Read the model definition and answer for the solid it produces. Units are mm, in the model's axes. Face numbers are marked on the shaded views. A direction names the side the tool comes from. Give positions to 0.01 mm unless a question says otherwise; leave off trailing zeros. Order: outer loops, then holes, each group sorted by start corner. A loop starts at its lowest first (then second) coordinate and runs counter-clockwise, first axis right, second up.
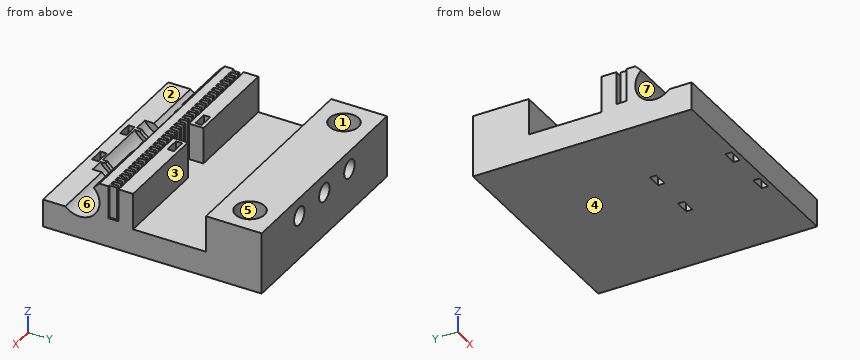
```python
from build123d import *

# Parameters (mm, degrees)
SKETCH1_W           = 60
SKETCH1_H           = 17
BOSS_EXTRUDE2_DEPTH = 60
SKETCH5_R           = 7.5
CUT_EXTRUDE3_DEPTH  = 12.5
BOSS_EXTRUDE5_START = 1
SKETCH7_R           = 7.5
SKETCH7_R_2         = 6.375
BOSS_EXTRUDE5_DEPTH = 1
SKETCH8_R           = 7.5
SKETCH8_R_2         = 6.375
BOSS_EXTRUDE6_DEPTH = 1
SKETCH3_W           = 14.616308542
SKETCH3_H           = 2.75
CUT_EXTRUDE2_DEPTH  = 87.539008545
SKETCH9_W           = 29.365083629
SKETCH9_H           = 1.75
SKETCH9_W_2         = 26.887211927
CUT_EXTRUDE4_DEPTH  = 4
SKETCH10_W          = 36.539507471
SKETCH10_H          = 1.75
SKETCH10_W_2        = 38.625095797
CUT_EXTRUDE5_DEPTH  = 4
SKETCH12_W          = 0.85
SKETCH12_H          = 2
BOSS_EXTRUDE7_DEPTH = 9
CUT_EXTRUDE6_DEPTH  = 10
SKETCH14_R          = 4
CUT_EXTRUDE7_DEPTH  = 15
SKETCH15_R          = 2.5
CUT_EXTRUDE8_DEPTH  = 15.3


with BuildPart() as part:
    # Sketch1 → Boss-Extrude2 (new body)
    with BuildSketch(Plane(origin=(0, 0, 0), x_dir=(1, 0, 0), z_dir=(0, 1, 0))):
        with Locations((30, 8.5)):
            Rectangle(SKETCH1_W, SKETCH1_H)
    extrude(amount=BOSS_EXTRUDE2_DEPTH)

    # Sketch5 → Cut-Extrude3 (cut, symmetric)
    with BuildSketch(Plane(origin=(30, 0, 0), x_dir=(0, 0, -1), z_dir=(1, 0, 0))):
        with Locations((5.5, 10)):
            Circle(SKETCH5_R)
    extrude(amount=CUT_EXTRUDE3_DEPTH, both=True, mode=Mode.SUBTRACT)

    # Sketch7 → Boss-Extrude5 (add)
    with BuildSketch(Plane(origin=(21.3, 0, 0), x_dir=(0, 0, -1), z_dir=(1, 0, 0)).offset(BOSS_EXTRUDE5_START)):
        with Locations((5.5, 10)):
            Circle(SKETCH7_R)
        with Locations((5.5, 10)):
            Circle(SKETCH7_R_2, mode=Mode.SUBTRACT)
    extrude(amount=-BOSS_EXTRUDE5_DEPTH)

    # Sketch8 → Boss-Extrude6 (add)
    with BuildSketch(Plane.ZY.offset(-38.7)):
        with Locations((-5.5, 10)):
            Circle(SKETCH8_R)
        with Locations(Location((-5.5, 10, 0), (0, 0, 180))):
            Circle(SKETCH8_R_2, mode=Mode.SUBTRACT)
    extrude(amount=BOSS_EXTRUDE6_DEPTH)

    # Sketch3 → Cut-Extrude2 (cut, through all)
    with BuildSketch(Plane(origin=(60, 0, 0), x_dir=(0, 0, -1), z_dir=(1, 0, 0))):
        with BuildLine():
            Line((0, 15.5), (-6.640665203, 15.5))
            Line((-6.640665203, 15.5), (-6.640665203, 0))
            Line((-6.640665203, 0), (0, 0))
            Line((0, 0), (9.389087297, 0))
            Line((9.389087297, 0), (9.389087297, 6.110912703))
            ThreePointArc((9.389087297, 6.110912703), (9.389087297, 13.889087297), (1.610912703, 13.889087297))
            Line((1.610912703, 13.889087297), (0, 15.5))
        make_face()
        with Locations((1.691845729, 19.325)):
            Rectangle(SKETCH3_W, SKETCH3_H)
    extrude(amount=-CUT_EXTRUDE2_DEPTH, mode=Mode.SUBTRACT)

    # Sketch9 → Cut-Extrude4 (cut)
    with BuildSketch(Plane(origin=(21.3, 0, 0), x_dir=(0, 0, -1), z_dir=(1, 0, 0))):
        with Locations((7.065771792, 2.125)):
            Rectangle(SKETCH9_W, SKETCH9_H)
        with Locations((6.15524604, 22.825)):
            Rectangle(SKETCH9_W_2, SKETCH9_H)
    extrude(amount=CUT_EXTRUDE4_DEPTH, mode=Mode.SUBTRACT)

    # Sketch10 → Cut-Extrude5 (cut)
    with BuildSketch(Plane.ZY.offset(-38.7)):
        with Locations((-12.469654385, 22.825)):
            Rectangle(SKETCH10_W, SKETCH10_H)
        with Locations((-10.676048425, 2.125)):
            Rectangle(SKETCH10_W_2, SKETCH10_H)
    extrude(amount=CUT_EXTRUDE5_DEPTH, mode=Mode.SUBTRACT)

    # Sketch12 → Boss-Extrude7 (add)
    with BuildSketch(Plane.XY.offset(-9)):
        with Locations((59.075, 18.95)):
            Rectangle(SKETCH12_W, SKETCH12_H)
        with Locations((57.075, 18.95)):
            Rectangle(SKETCH12_W, SKETCH12_H)
        with Locations((55.075, 18.95)):
            Rectangle(SKETCH12_W, SKETCH12_H)
        with Locations((53.075, 18.95)):
            Rectangle(SKETCH12_W, SKETCH12_H)
        with Locations((51.075, 18.95)):
            Rectangle(SKETCH12_W, SKETCH12_H)
        with Locations((49.075, 18.95)):
            Rectangle(SKETCH12_W, SKETCH12_H)
        with Locations((47.075, 18.95)):
            Rectangle(SKETCH12_W, SKETCH12_H)
        with Locations((45.075, 18.95)):
            Rectangle(SKETCH12_W, SKETCH12_H)
        with Locations((43.075, 18.95)):
            Rectangle(SKETCH12_W, SKETCH12_H)
        with Locations((41.075, 18.95)):
            Rectangle(SKETCH12_W, SKETCH12_H)
        with Locations((39.075, 18.95)):
            Rectangle(SKETCH12_W, SKETCH12_H)
        with Locations((37.075, 18.95)):
            Rectangle(SKETCH12_W, SKETCH12_H)
        with Locations((35.075, 18.95)):
            Rectangle(SKETCH12_W, SKETCH12_H)
        with Locations((33.075, 18.95)):
            Rectangle(SKETCH12_W, SKETCH12_H)
        with Locations((31.075, 18.95)):
            Rectangle(SKETCH12_W, SKETCH12_H)
        with Locations((29.075, 18.95)):
            Rectangle(SKETCH12_W, SKETCH12_H)
        with Locations((27.075, 18.95)):
            Rectangle(SKETCH12_W, SKETCH12_H)
        with Locations((25.075, 18.95)):
            Rectangle(SKETCH12_W, SKETCH12_H)
        with Locations((23.075, 18.95)):
            Rectangle(SKETCH12_W, SKETCH12_H)
        with Locations((21.075, 18.95)):
            Rectangle(SKETCH12_W, SKETCH12_H)
        with Locations((19.075, 18.95)):
            Rectangle(SKETCH12_W, SKETCH12_H)
        with Locations((17.075, 18.95)):
            Rectangle(SKETCH12_W, SKETCH12_H)
        with Locations((15.075, 18.95)):
            Rectangle(SKETCH12_W, SKETCH12_H)
        with Locations((13.075, 18.95)):
            Rectangle(SKETCH12_W, SKETCH12_H)
        with Locations((11.075, 18.95)):
            Rectangle(SKETCH12_W, SKETCH12_H)
        with Locations((9.075, 18.95)):
            Rectangle(SKETCH12_W, SKETCH12_H)
        with Locations((7.075, 18.95)):
            Rectangle(SKETCH12_W, SKETCH12_H)
        with Locations((5.075, 18.95)):
            Rectangle(SKETCH12_W, SKETCH12_H)
        with Locations((3.075, 18.95)):
            Rectangle(SKETCH12_W, SKETCH12_H)
        with Locations((1.075, 18.95)):
            Rectangle(SKETCH12_W, SKETCH12_H)
    extrude(amount=BOSS_EXTRUDE7_DEPTH)

    # Sketch13 → Cut-Extrude6 (cut)
    with BuildSketch(Plane.XY):
        Polygon((33.7, 24.7), (33.7, 20.7), (26.3, 20.7), (26.3, 24.7), (-1.390912484, 24.7), (-1.390912484, 44.7), (62.591854088, 44.7), (62.591854088, 24.7), align=None)
    extrude(amount=-CUT_EXTRUDE6_DEPTH, mode=Mode.SUBTRACT)

    # Sketch14 → Cut-Extrude7 (cut)
    with BuildSketch(Plane.XY):
        with Locations((7.5, 52.5)):
            Circle(SKETCH14_R)
        with Locations((52.5, 52.5)):
            Circle(SKETCH14_R)
    extrude(amount=-CUT_EXTRUDE7_DEPTH, mode=Mode.SUBTRACT)

    # Sketch15 → Cut-Extrude8 (cut)
    with BuildSketch(Plane.XZ.offset(-44.7)):
        with Locations(Location((30, -5, 0), (0, 0, 270))):
            Circle(SKETCH15_R)
        with Locations(Location((18, -5, 0), (0, 0, 270))):
            Circle(SKETCH15_R)
        with Locations(Location((42, -5, 0), (0, 0, 270))):
            Circle(SKETCH15_R)
    extrude(amount=-CUT_EXTRUDE8_DEPTH, mode=Mode.SUBTRACT)


solid = part.part
```
1) The part is cut by section C-C on z = -5. Count the separate pieces of the cut face and the enclosed holes in it, and give its area (3 significant figures).
Final values:
separate pieces: 7
enclosed holes: 4
area: 936 mm2
2) Consider L1, parallel to X at y = 52.75, z = -5; L2, parallel to Y at x = 49, z = -7; L3, parallel to X at y = 54.5, z = -5. Determine where each line is inside the solid, lowest interval first.
Final values:
L1: x = 0 to 3.51, 11.49 to 15.5, 20.5 to 27.5, 32.5 to 39.5, 44.5 to 48.51, 56.49 to 60
L2: y = 15.29 to 19.95, 20.7 to 24.7, 44.7 to 50.56, 54.44 to 60
L3: x = 0 to 4.04, 10.96 to 15.5, 20.5 to 27.5, 32.5 to 39.5, 44.5 to 49.04, 55.96 to 60
3) Given pin 1 (1.5 mm diameter, centred on y = 25, z = -2, fed in from -X); pin 2 (2 mm diameter, centred on y = 42.5, z = -3.5, fed in from +X); pin 3 (1.6 mm diameter, centred on y = 19, z = -2.5, fed in from +X); pin 4 (1 mm diameter, centred on y = 19, z = -3, fed in from -X), each flat-ended and moving along its own axis, determine where each tip first touches the part or whether it passes through.
Final values:
pin 1: stops at x = 0
pin 2: passes through
pin 3: stops at x = 59.5
pin 4: stops at x = 0.65
4) The part is cut by section B-B on y = 10. Determine the outline of the cut face in (x, z) (3 decimals), and give its area (3 significant figures).
Final values:
outline: (0, -17) - (60, -17) - (60, -11) - (42.5, -11) - (42.5, -13) - (38.7, -13) - (38.7, -11.875) - (37.7, -11.875) - (37.7, -13) - (22.3, -13) - (22.3, -11.875) - (21.3, -11.875) - (21.3, -13) - (17.5, -13) - (17.5, -11) - (0, -11) - close
area: 312 mm2
5) The part is cut by section D-D on y = 43. Determine the outline of the cut face in (x, z), and give its area (3 significant figures).
Final values:
outline: (0, -17) - (60, -17) - (60, -10) - (0, -10) - close
area: 420 mm2
6) A tool of negligible diameter and unlimited length cuts with its end or side. For the marked faces 1, 2 and 3, from which of +Z, -Z, +X, -X, +Y, -Y can it reach the whole face along a straight path? Write none if from no direction.
Final values:
face 1: +Z
face 2: +Z, +X, -X, -Y
face 3: +Z, +X, -X
7) For a pull along Z with two mould halves and no side action, classify the marked faces 4, 5, 6 and 7 as released by +Z, released by -Z, zero draft, split by the parting line, or undercut.
Final values:
face 4: released by -Z
face 5: zero draft
face 6: undercut
face 7: undercut
8) The part is cut by section A-A on y = 52.5. Determine the outline of the cut face in (x, z), and give its area (3 significant figures).
Final values:
outline: (0, -17) - (60, -17) - (60, 0) - (56.5, 0) - (56.5, -15) - (48.5, -15) - (48.5, 0) - (11.5, 0) - (11.5, -15) - (3.5, -15) - (3.5, 0) - (0, 0) - close; hole circle Ø5 at (18, -5); hole circle Ø5 at (30, -5); hole circle Ø5 at (42, -5)
area: 721 mm2
